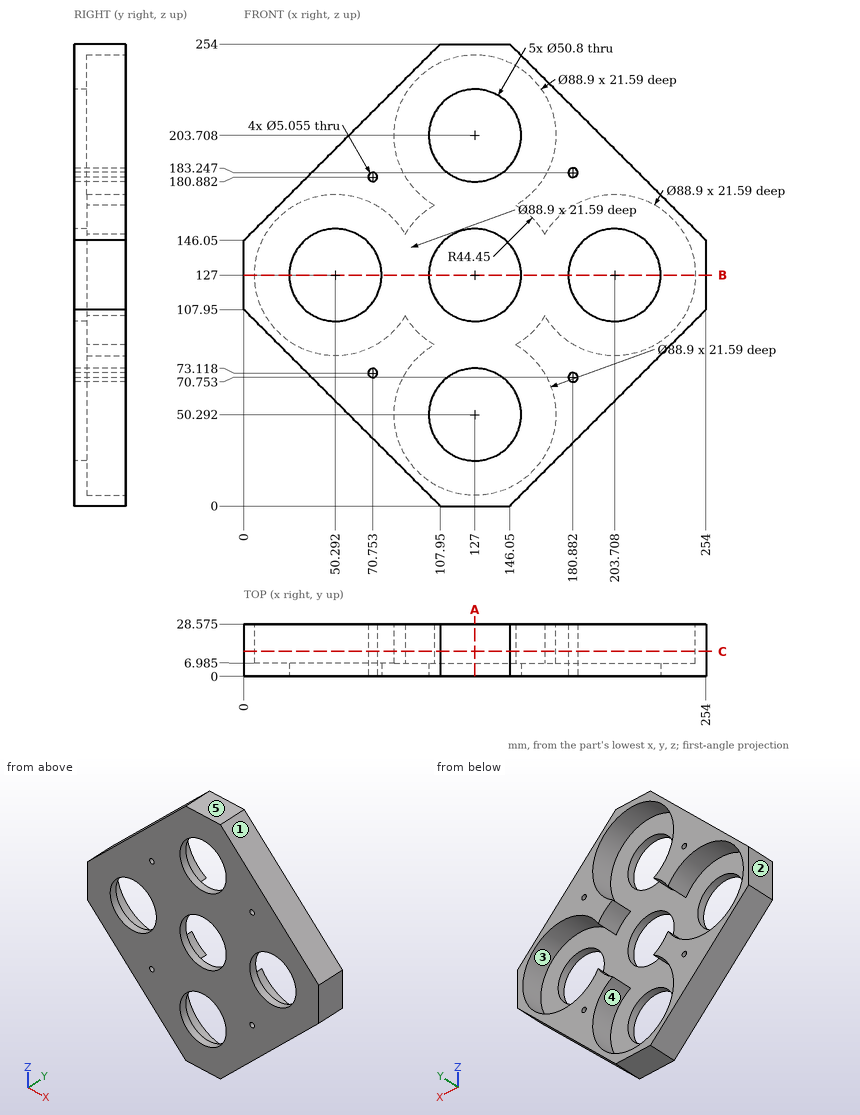
The figure shows three views and two pictorial views of one solid part (mm, origin at its lowest corner). Answer the questions. A direction names the side the tool comes from. Coordinates: 2 decimals unless noted, no trailing zeros. Loops run counter-clockwise (first coordinate to the right, second up) from the corner with the lowest first, then second, coordinate; pieces in that order, holes last. Notation, with made-up numbers: (33.25, -28) - (58.25, -28) arc R24 cw to (58.25, -18) - close; hole circle Ø1 at (12.25, 24.25). An arc over 180 degrees is marked (long way). Use a Markdown table: item, result. Add a question column.
1) Find the intervals of material crossed by line 1 (Z direction, x = 127, y = 1.75); line 2 (Z direction, x = 127, y = 23.5); line 3 (Z direction, x = 124.5, y = 1.75) (1 decimal), in increasing order.
2) The mould has two halves that part along Z. Classify the marked faces 1, 2 and 3: released by +Z, released by -Z, zero draft, split by the parting line, or undercut.
3) The part is cut by section C-C, the plane y = 13.5. State how many separate pieces and enclosed holes the cut face has, and give its area (3 significant figures).
4) Given pin 1 (4 mm diameter, centred on x = 180.88, z = 183.25, fed in from +Y); pin 2 (8 mm diameter, centred on x = 180.88, z = 70.75, fed in from -Y); pin 3 (3 mm diameter, centred on x = 43, y = 11, fed in from +Z); pin 4 (4 mm diameter, centred on x = 189, y = 9.5, fed in from -Z), each flat-ended and moving along its own axis, determine where each tip first touches the part or whether it passes through.
5) The part is cut by section B-B, the plane z = 127. Give the vertices of the cut face in (x, y) (1 decimal), and give its area (3 significant figures).
6) For the marked faces 4 and 5, determine the directions among +Z, -Z, +X, -X, +Y, -Y from which every point of the face is accessible in a straight line to the end or side of a thin tool.
7) The part is cut by section A-A, the plane x = 127. Give the vertices of the cut face in (y, z) (1 decimal).
Here are the results:
| question | item | result |
|---|---|---|
| 1 | line 1 | z = 0 to 24.89, 75.69 to 101.6, 152.4 to 178.31, 229.11 to 254 |
| 1 | line 2 | z = 0 to 5.84, 248.16 to 254 |
| 1 | line 3 | z = 0 to 25, 75.6 to 101.7, 152.3 to 178.4, 229 to 254 |
| 2 | face 1 | released by +Z |
| 2 | face 2 | zero draft |
| 2 | face 3 | undercut |
| 3 | separate pieces | 1 |
| 3 | enclosed holes | 5 |
| 3 | area | 11,600 mm^2 |
| 4 | pin 1 | passes through |
| 4 | pin 2 | stops at y = 0 |
| 4 | pin 3 | stops at z = 190.55 |
| 4 | pin 4 | stops at z = 40.95 |
| 5 | outline | (0, 0) - (24.9, 0) - (24.9, 7) - (5.8, 7) - (5.8, 28.6) - (0, 28.6) - close; (75.7, 0) - (101.6, 0) - (101.6, 7) - (75.7, 7) - close; (152.4, 0) - (178.3, 0) - (178.3, 7) - (152.4, 7) - close; (229.1, 0) - (254, 0) - (254, 28.6) - (248.2, 28.6) - (248.2, 7) - (229.1, 7) - close |
| 5 | area | 962 mm^2 |
| 6 | face 4 | +Y |
| 6 | face 5 | +Z, +X, -X, +Y, -Y |
| 7 | outline | (0, 0) - (28.6, 0) - (28.6, 5.8) - (7, 5.8) - (7, 24.9) - (0, 24.9) - close; (0, 75.7) - (7, 75.7) - (7, 101.6) - (0, 101.6) - close; (0, 152.4) - (7, 152.4) - (7, 178.3) - (0, 178.3) - close; (0, 229.1) - (7, 229.1) - (7, 248.2) - (28.6, 248.2) - (28.6, 254) - (0, 254) - close |
